Geometry check sheet. Reference: the model listing, model coordinates, mm. Face numbers are marked on the shaded views. A direction names the side the tool comes from. Round coordinates to 2 decimals unless told otherwise and drop trailing zeros. Order: outer loops, then holes, each group sorted by start corner. A loop starts at its lowest first (then second) coordinate and runs counter-clockwise, first axis right, second up.
(1) Set-up check for the marked faces 4 and 5: record each of +Z, -Z, +X, -X, +Y, -Y from which the full face is reachable in a straight line by a thin tool's end or side.
(2) Draft check along X on the marked faces 1, 2 and 3. Enter one of: pulls with the +X half, pulls with the -X half, needs draft (parallel to the pull), parting line crosses it, or undercut.
(3) Cross-section at B-B on z = 8. Enter the section's corners in (x, y).
(4) Thickness scan on L1, parallel to X at y = -21, z = 17.5; L2, parallel to X at y = -30.5, z = 19.5; L3, parallel to Y at x = 50, z = 22.25. Record the ranges inside material, lowest first.
(5) Gauge pin test, flat ends, axial feed: P1, Ø8, axis at x = 64, z = 8.5, coming from the +Y side; P2, Ø1.5, axis at x = 56.5, y = -27, coming from the -Z side. Record the tip position at first contact, or that the pin passes through.
(6) Cross-section at A-A on y = -29.5. Enter the section's corners in (x, z).
(7) Cross-section at D-D on y = -24. Enter the section's corners in (x, z), and give its area (3 significant figures).
(8) Cross-section at C-C on x = 51. Enter the section's corners in (y, z), and give its area (3 significant figures).
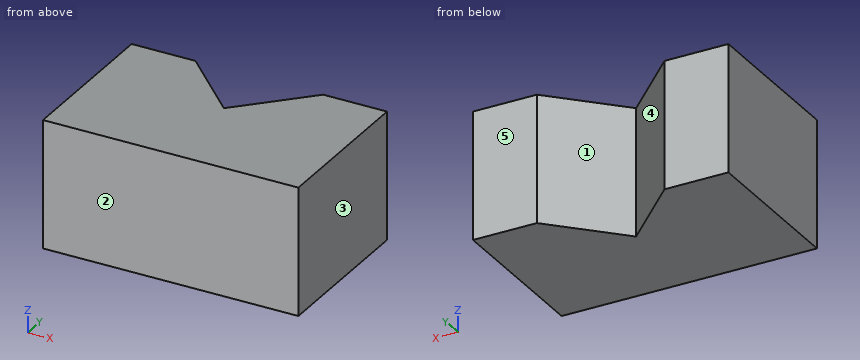
from build123d import *

# Parameters (mm, degrees)
F0_W     = 50.8
F0_H     = 6.35
F1_DEPTH = 25.4
F3_DEPTH = 25.4
F5_DEPTH = 25.4
F7_DEPTH = 25.4


with BuildPart() as f1:
    # F0 (on Top) → F1 (new body)
    with BuildSketch(Plane.XY):
        with Locations((59.120102, -48.131117)):
            Rectangle(F0_W, F0_H)
    extrude(amount=F1_DEPTH)

    # F2 (on face) → F3 (join)
    with BuildSketch(Plane.XY.offset(25.4)):
        Polygon((59.120102, -44.956117), (84.520102, -44.956117), (84.520102, -19.556117), align=None)
    extrude(amount=-F3_DEPTH)

    # F4 (on face) → F5 (join)
    with BuildSketch(Plane.XY.offset(25.4)):
        Polygon((33.720102, -19.556117), (33.720102, -44.956117), (59.120102, -44.956117), align=None)
    extrude(amount=-F5_DEPTH)

    # F6 (on face) → F7 (join)
    with BuildSketch(Plane(origin=(0, 0, 0), x_dir=(1, 0, 0), z_dir=(0, 0, -1))):
        Polygon((71.820102, 19.556117), (84.520102, 19.556117), (59.120102, 44.956117), (33.720102, 19.556117), (46.420102, 19.556117), (59.120102, 32.252281), align=None)
    extrude(amount=-F7_DEPTH)


solid = f1.part
Found:
1. face 4: +Z, -Z, +Y
1. face 5: +Z, -Z, +X, -X, +Y
2. face 1: undercut
2. face 2: needs draft
2. face 3: pulls with the +X half
3. outline: (33.72, -51.31) - (84.52, -51.31) - (84.52, -19.56) - (71.82, -19.56) - (59.12, -32.25) - (46.42, -19.56) - (33.72, -19.56) - close
4. L1: x = 33.72 to 47.86, 70.38 to 84.52
4. L2: x = 33.72 to 57.37, 60.87 to 84.52
4. L3: y = -51.31 to -23.13
5. P1: stops at y = -23.38
5. P2: passes through
6. outline: (33.72, 0) - (56.37, 0) - (56.37, 25.4) - (33.72, 25.4) - close; (61.87, 0) - (84.52, 0) - (84.52, 25.4) - (61.87, 25.4) - close
7. outline: (33.72, 0) - (50.87, 0) - (50.87, 25.4) - (33.72, 25.4) - close; (67.37, 0) - (84.52, 0) - (84.52, 25.4) - (67.37, 25.4) - close
7. area: 871 mm2
8. outline: (-51.31, 0) - (-24.13, 0) - (-24.13, 25.4) - (-51.31, 25.4) - close
8. area: 690 mm2
